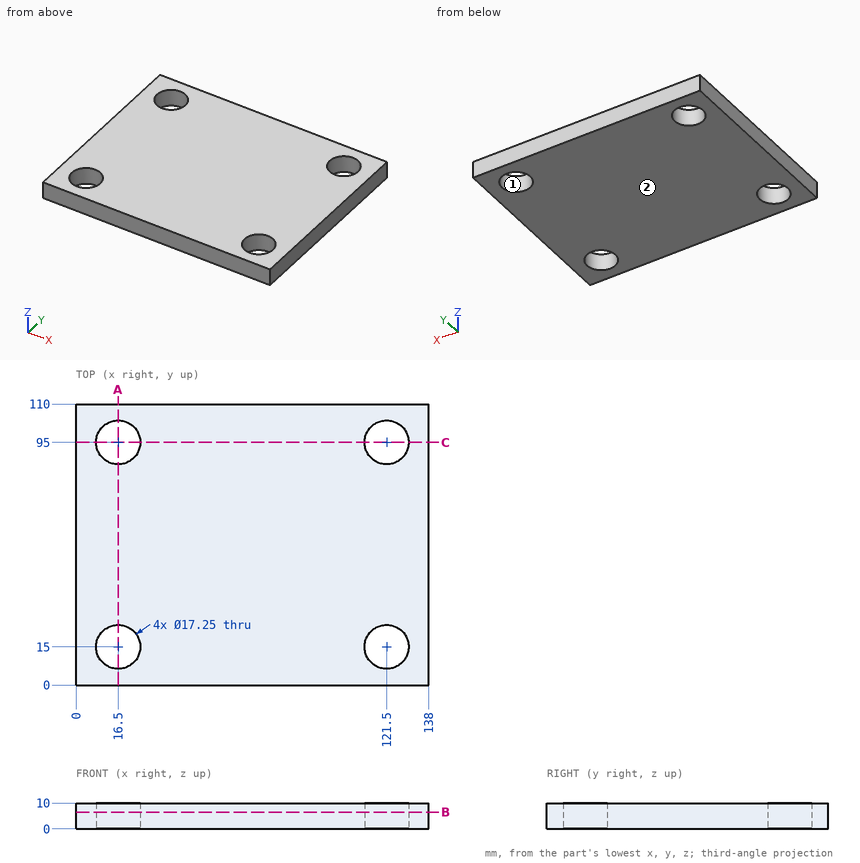
Check sheet for the drawn part. Datum: minimum x, y, z corner. Units: mm. Give positions to 0.01 mm unless a question says otherwise; leave off trailing zeros. Order: outer loops, then holes, each group sorted by start corner. A loop starts at its lowest first (then second) coordinate and runs counter-clockwise, first axis right, second up. Notation, with made-up numbers: (78, 23) - (89, 23) arc R12 ccw to (89, 46) - close; hole circle Ø2 at (8, -19.75). An arc over 180 degrees is marked (long way). Write item = value, one per line. Start each with the question number.
1) Section check C-C (y = 95). Enter the section's corners in (x, z) (3 decimals), then the cut area to 4 significant figures.
2) Draft check along X on the marked faces 1 and 2. Enter one of: released by +X, released by -X, zero draft, split by the parting line, or undercut.
3) Section check A-A (x = 16.5). Enter the section's corners in (y, z) (3 decimals), then the cut area to 3 significant figures.
4) Gauge pin test, flat ends, axial feed: pin 1 Ø12 at (x, y) = (115.5, 19) entering from -Z; pin 2 Ø10.5 at (x, y) = (16.5, 95) entering from +Z. Record the tip position at first contact, or that the pin passes through.
5) Scan lines: L1, parallel to Y at x = 16.5, z = 6.75 (3 decimals); L2, parallel to X at y = 95, z = 5.5 (3 decimals); L3, parallel to Y at x = 118, z = 5.5. Record each from-to range of solid material in increasing order.
6) Section check B-B (z = 6.5). Enter the section's corners in (x, y) (3 decimals).
Geometry check:
q1.outline = (0, 0) - (7.875, 0) - (7.875, 10) - (0, 10) - close; (25.125, 0) - (112.875, 0) - (112.875, 10) - (25.125, 10) - close; (130.125, 0) - (138, 0) - (138, 10) - (130.125, 10) - close
q1.area = 1,035 mm2
q2.face_1 = undercut
q2.face_2 = zero draft
q3.outline = (0, 0) - (6.375, 0) - (6.375, 10) - (0, 10) - close; (23.625, 0) - (86.375, 0) - (86.375, 10) - (23.625, 10) - close; (103.625, 0) - (110, 0) - (110, 10) - (103.625, 10) - close
q3.area = 755 mm2
q4.pin_1 = 0
q4.pin_2 = through
q5.L1 = 0 to 6.375, 23.625 to 86.375, 103.625 to 110
q5.L2 = 0 to 7.875, 25.125 to 112.875, 130.125 to 138
q5.L3 = 0 to 7.12, 22.88 to 87.12, 102.88 to 110
q6.outline = (0, 0) - (138, 0) - (138, 110) - (0, 110) - close; hole circle Ø17.25 at (16.5, 15); hole circle Ø17.25 at (16.5, 95); hole circle Ø17.25 at (121.5, 15); hole circle Ø17.25 at (121.5, 95)
